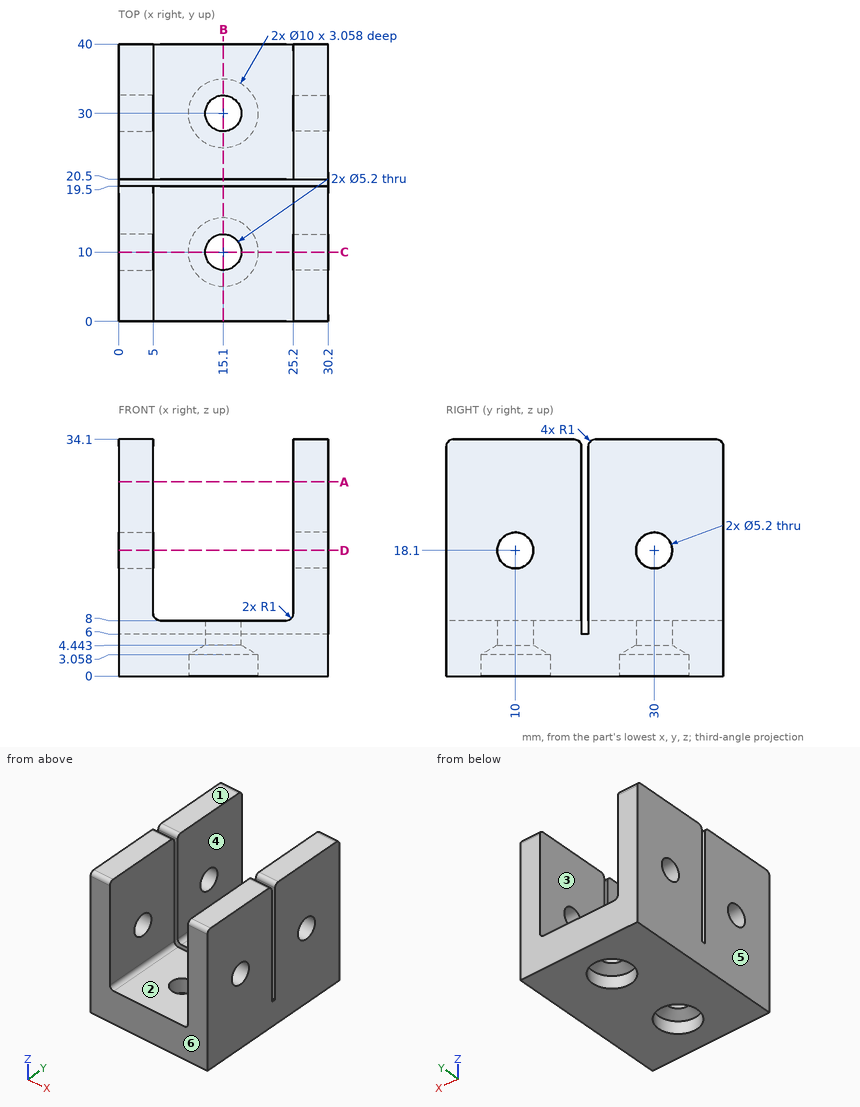
Geometry check sheet. Reference: drawing and pictorial views, mm from the part's lowest x, y, z. A direction names the side the tool comes from. Round coordinates to 2 decimals unless told otherwise and drop trailing zeros. Order: outer loops, then holes, each group sorted by start corner. A loop starts at its lowest first (then second) coordinate and runs counter-clockwise, first axis right, second up. Notation, with made-up numbers: (52, 64.25) - (104, 64.25) arc R37 cw to (104, 101.25) - close; hole circle Ø10 at (-10, 18). An arc over 180 degrees is marked (long way). Use a Markdown table: item, result. Add a question column.
1) Set-up check for the marked faces 1 and 2: record each of +Z, -Z, +X, -X, +Y, -Y from which the full face is reachable in a straight line by a thin tool's end or side.
2) Thickness scan on line 1 along Y through (x, z) = (15.1, 2.2); line 2 along Y through (x, z) = (28, 18); line 3 along X through (y, z) = (18, 15). Record the ranges inside material, lowest first.
3) Section check D-D (z = 18.1). Count the separate pieces of the cut face and the enclosed holes in it, then the cut area to 3 significant figures.
4) Section check C-C (y = 10). Record the cut outline in (x, z).
5) Section check A-A (z = 28). Record the cut outline in (x, y), then the cut area to 3 significant figures.
6) Section check B-B (x = 15.1). Record the cut outline in (y, z).
7) Gauge pin test, flat ends, axial feed: P1, Ø14.5, axis at x = 12.5, y = 12, coming from the +Z side; P2, Ø0.8, axis at x = 14.5, y = 20, coming from the +Z side; P3, Ø6, axis at x = 15.1, y = 10, coming from the +Z side. Record the tip position at first contact, or that the pin passes through.
8) Mould release check, pull along X, two halves, no side actions. Record for the marked faces 3, 4, 5 and 6: released by +X, released by -X, zero draft, split by the parting line, or undercut.
Established:
| question | item | result |
|---|---|---|
| 1 | face 1 | +Z, +X, -X, +Y, -Y |
| 1 | face 2 | +Z, +Y, -Y |
| 2 | line 1 | 0 to 5, 15 to 25, 35 to 40 |
| 2 | line 2 | 0 to 7.4, 12.6 to 19.5, 20.5 to 27.4, 32.6 to 40 |
| 2 | line 3 | 0 to 5, 25.2 to 30.2 |
| 3 | separate pieces | 8 |
| 3 | enclosed holes | 0 |
| 3 | area | 286 mm2 |
| 4 | outline | (0, 0) - (10.1, 0) - (10.1, 3.06) - (12.5, 4.44) - (12.5, 8) - (6, 8) arc R1 cw to (5, 9) - (5, 15.5) - (0, 15.5) - close; (0, 20.7) - (5, 20.7) - (5, 34.1) - (0, 34.1) - close; (17.7, 4.44) - (20.1, 3.06) - (20.1, 0) - (30.2, 0) - (30.2, 15.5) - (25.2, 15.5) - (25.2, 9) arc R1 cw to (24.2, 8) - (17.7, 8) - close; (25.2, 20.7) - (30.2, 20.7) - (30.2, 34.1) - (25.2, 34.1) - close |
| 5 | outline | (0, 0) - (5, 0) - (5, 19.5) - (0, 19.5) - close; (0, 20.5) - (5, 20.5) - (5, 40) - (0, 40) - close; (25.2, 0) - (30.2, 0) - (30.2, 19.5) - (25.2, 19.5) - close; (25.2, 20.5) - (30.2, 20.5) - (30.2, 40) - (25.2, 40) - close |
| 5 | area | 390 mm2 |
| 6 | outline | (0, 0) - (5, 0) - (5, 3.06) - (7.4, 4.44) - (7.4, 8) - (0, 8) - close; (12.6, 4.44) - (15, 3.06) - (15, 0) - (25, 0) - (25, 3.06) - (27.4, 4.44) - (27.4, 8) - (20.5, 8) - (20.5, 6) - (19.5, 6) - (19.5, 8) - (12.6, 8) - close; (32.6, 4.44) - (35, 3.06) - (35, 0) - (40, 0) - (40, 8) - (32.6, 8) - close |
| 7 | P1 | z = 8.34 |
| 7 | P2 | z = 6 |
| 7 | P3 | z = 8 |
| 8 | face 3 | undercut |
| 8 | face 4 | undercut |
| 8 | face 5 | released by -X |
| 8 | face 6 | zero draft |
